Here's how the part is built. I have some questions about the finished solid (model axes, mm). Face numbers are marked on the shaded views. A direction names the side the tool comes from. Give positions to 0.01 mm unless a question says otherwise; leave off trailing zeros. Loops run counter-clockwise (first coordinate to the right, second up) from the corner with the lowest first, then second, coordinate; pieces in that order, holes last. Notation, with made-up numbers: (56, -26.75) - (109, -26.75) arc R36 cw to (109, 7.25) - close; hole circle Ø4 at (13.25, 10). An arc over 180 degrees is marked (long way). Return JSON: item names as keys, results as strings. Group by question number.
(1) I need wall thicknesses on probe 1 along X at (y, z) = (20, 17); probe 2 along X at (y, z) = (52, 0); probe 3 along Y at (x, z) = (-4.5, -24). Which ranges of each line are inside material? Lowest first, please. Write a range as [from, to].
(2) For P1, Ø3.5, axis at x = 0.5, y = 47.5, coming from the -Z side; P2, Ø6, axis at x = 5.5, z = -25.5, coming from the -Y side; P3, Ø4, axis at x = -14.5, y = 11.5, coming from the -Z side, each with a flat end and sliding along its axis, tell me the tip position at first contact or that it passes through.
(3) If we section it at C-C (y = 32): Please give me the cut outline in (x, z).
(4) If we mould it in two halves opening along Z, with no side actions, what happens to the marked faces 1, 2, 3 and 4? For each: released by +Z, released by -Z, zero draft, split by the parting line, or undercut.
(5) If we section it at A-A (x = -1.5): Please give me the cut outline in (y, z).
(6) If we section it at B-B (z = 16): Please give me the cut outline in (x, y), then the cut area to 3 significant figures.
(7) If we section it at D-D (y = 71): Please give me the cut outline in (x, z), then the cut area to 3 significant figures.
(8) On a 3-axis mill with a long thin cutter (end or side, diameter ignored), from which of +Z, -Z, +X, -X, +Y, -Y can I reach the whole of each face in a straight line? I mean the marked faces 5, 6, 7, 8 and 9. Say none if no direction works.
```python
from build123d import *

# Parameters (mm, degrees)
SKETCH1_W               = 49
SKETCH1_H               = 49
SKETCH1_R               = 3.25
BOSS_EXTRUDE1_DEPTH     = 53
SKETCH2_W               = 44
SKETCH2_H               = 44
CUT_EXTRUDE1_DEPTH      = 47
SKETCH3_R               = 13
CUT_EXTRUDE2_DEPTH      = 2
CUT_EXTRUDE3_DEPTH      = 10
BOSS_EXTRUDE2_DEPTH     = 30
SKETCH7_W               = 20.5
SKETCH7_H               = 21
CUT_EXTRUDE6_DEPTH      = 59
CUT_EXTRUDE7_DEPTH      = 59
CUT_EXTRUDE7_DEPTH_BACK = 3
SKETCH10_R              = 2.75
CUT_EXTRUDE8_DEPTH      = 59
FILLET1_R               = 30
CUT_EXTRUDE9_DEPTH      = 50.0000001


with BuildPart() as part:
    # Sketch1 → Boss-Extrude1 (new body)
    with BuildSketch(Plane(origin=(0, 0, 0), x_dir=(1, 0, 0), z_dir=(0, 1, 0))):
        Rectangle(SKETCH1_W, SKETCH1_H)
        Circle(SKETCH1_R, mode=Mode.SUBTRACT)
    extrude(amount=BOSS_EXTRUDE1_DEPTH)

    # Sketch2 → Cut-Extrude1 (cut)
    with BuildSketch(Plane.XZ):
        Rectangle(SKETCH2_W, SKETCH2_H)
    extrude(amount=-CUT_EXTRUDE1_DEPTH, mode=Mode.SUBTRACT)

    # Sketch3 → Cut-Extrude2 (cut)
    with BuildSketch(Plane.XZ.offset(-47)):
        Circle(SKETCH3_R)
    extrude(amount=-CUT_EXTRUDE2_DEPTH, mode=Mode.SUBTRACT)

    # Sketch4 → Cut-Extrude3 (cut)
    with BuildSketch(Plane(origin=(0, 53, 0), x_dir=(1, 0, 0), z_dir=(0, 1, 0))):
        with BuildLine():
            Line((-14.86862915, 17.13137085), (-11.36862915, 13.63137085))
            ThreePointArc((-11.36862915, 13.63137085), (-11.36862915, 11.36862915), (-13.63137085, 11.36862915))
            Line((-13.63137085, 11.36862915), (-17.13137085, 14.86862915))
            ThreePointArc((-17.13137085, 14.86862915), (-17.13137085, 17.13137085), (-14.86862915, 17.13137085))
        make_face()
        with BuildLine():
            Line((11.36862915, 13.63137085), (14.86862915, 17.13137085))
            ThreePointArc((14.86862915, 17.13137085), (17.13137085, 17.13137085), (17.13137085, 14.86862915))
            Line((17.13137085, 14.86862915), (13.63137085, 11.36862915))
            ThreePointArc((13.63137085, 11.36862915), (11.36862915, 11.36862915), (11.36862915, 13.63137085))
        make_face()
        with BuildLine():
            Line((13.63137085, -11.36862915), (17.13137085, -14.86862915))
            ThreePointArc((17.13137085, -14.86862915), (17.13137085, -17.13137085), (14.86862915, -17.13137085))
            Line((14.86862915, -17.13137085), (11.36862915, -13.63137085))
            ThreePointArc((11.36862915, -13.63137085), (11.36862915, -11.36862915), (13.63137085, -11.36862915))
        make_face()
        with BuildLine():
            Line((-11.36862915, -13.63137085), (-14.86862915, -17.13137085))
            ThreePointArc((-14.86862915, -17.13137085), (-17.13137085, -17.13137085), (-17.13137085, -14.86862915))
            Line((-17.13137085, -14.86862915), (-13.63137085, -11.36862915))
            ThreePointArc((-13.63137085, -11.36862915), (-11.36862915, -11.36862915), (-11.36862915, -13.63137085))
        make_face()
    extrude(amount=-CUT_EXTRUDE3_DEPTH, mode=Mode.SUBTRACT)

    # Sketch5 → Boss-Extrude2 (add)
    with BuildSketch(Plane(origin=(0, 53, 0), x_dir=(1, 0, 0), z_dir=(0, 1, 0))):
        with BuildLine():
            Line((-20.5, -24.5), (-12.942531675, 1.221013453))
            ThreePointArc((-12.942531675, 1.221013453), (-8.750052146, 9.614394804), (0, 13))
            ThreePointArc((0, 13), (8.750052146, 9.614394804), (12.942531675, 1.221013453))
            Line((12.942531675, 1.221013453), (20.5, -24.5))
            Line((20.5, -24.5), (24.5, -24.5))
            Line((24.5, -24.5), (24.5, 35))
            Line((24.5, 35), (-24.5, 35))
            Line((-24.5, 35), (-24.5, -24.5))
            Line((-24.5, -24.5), (-20.5, -24.5))
        make_face()
    extrude(amount=BOSS_EXTRUDE2_DEPTH)

    # Sketch7 → Cut-Extrude6 (cut)
    with BuildSketch(Plane.ZY.offset(24.5)):
        with Locations((-24.75, 63.5)):
            Rectangle(SKETCH7_W, SKETCH7_H)
    extrude(amount=-CUT_EXTRUDE6_DEPTH, mode=Mode.SUBTRACT)

    # Sketch9 → Cut-Extrude7 (cut, two sides)
    with BuildSketch(Plane(origin=(0, 53, 0), x_dir=(1, 0, 0), z_dir=(0, 1, 0))) as cut_extrude7_sk:
        with BuildLine():
            Line((-14.621320344, 10.378679656), (-18.121320344, 13.878679656))
            ThreePointArc((-18.121320344, 13.878679656), (-18.121320344, 18.121320344), (-13.878679656, 18.121320344))
            Line((-13.878679656, 18.121320344), (-10.378679656, 14.621320344))
            ThreePointArc((-10.378679656, 14.621320344), (-10.378679656, 10.378679656), (-14.621320344, 10.378679656))
        make_face()
        with BuildLine():
            Line((10.378679656, 14.621320344), (13.878679656, 18.121320344))
            ThreePointArc((13.878679656, 18.121320344), (18.121320344, 18.121320344), (18.121320344, 13.878679656))
            Line((18.121320344, 13.878679656), (14.621320344, 10.378679656))
            ThreePointArc((14.621320344, 10.378679656), (10.378679656, 10.378679656), (10.378679656, 14.621320344))
        make_face()
        with BuildLine():
            Line((13.878679656, -18.121320344), (10.378679656, -14.621320344))
            ThreePointArc((10.378679656, -14.621320344), (10.378679656, -10.378679656), (14.621320344, -10.378679656))
            Line((14.621320344, -10.378679656), (18.121320344, -13.878679656))
            ThreePointArc((18.121320344, -13.878679656), (18.121320344, -18.121320344), (13.878679656, -18.121320344))
        make_face()
        with BuildLine():
            Line((-13.878679656, -18.121320344), (-10.378679656, -14.621320344))
            ThreePointArc((-10.378679656, -14.621320344), (-10.378679656, -10.378679656), (-14.621320344, -10.378679656))
            Line((-14.621320344, -10.378679656), (-18.121320344, -13.878679656))
            ThreePointArc((-18.121320344, -13.878679656), (-18.121320344, -18.121320344), (-13.878679656, -18.121320344))
        make_face()
    extrude(amount=CUT_EXTRUDE7_DEPTH, mode=Mode.SUBTRACT)
    extrude(cut_extrude7_sk.sketch, amount=-CUT_EXTRUDE7_DEPTH_BACK, mode=Mode.SUBTRACT)

    # Sketch10 → Cut-Extrude8 (cut)
    with BuildSketch(Plane.XZ.offset(-74)):
        with Locations((14.5, -24.5)):
            Circle(SKETCH10_R)
        with Locations((-14.5, -24.5)):
            Circle(SKETCH10_R)
    extrude(amount=-CUT_EXTRUDE8_DEPTH, mode=Mode.SUBTRACT)

    # Fillet1
    fillet1_edges = [part.edges().sort_by_distance(p)[0] for p in [
        (22.5, 83, 24.5),
        (-22.5, 83, 24.5),
    ]]
    fillet(fillet1_edges, radius=FILLET1_R)

    # Sketch11 → Cut-Extrude9 (cut, through all)
    with BuildSketch(Plane(origin=(24.5, 0, 0), x_dir=(0, 0, -1), z_dir=(1, 0, 0))):
        Polygon((24.5, 0), (24.5, 42), (22, 42), (-22, 0), align=None)
    extrude(amount=-CUT_EXTRUDE9_DEPTH, mode=Mode.SUBTRACT)


solid = part.part
```
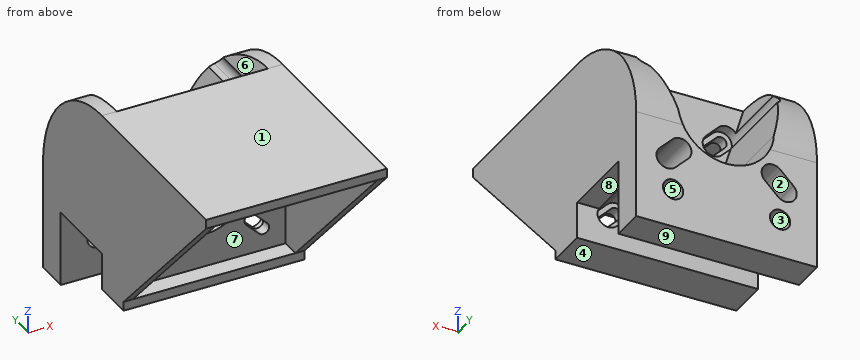
Values:
{
 "1": {"probe 1": "[-24.5, -22], [22, 24.5]", "probe 2": "[-24.5, -3.25], [3.25, 24.5]", "probe 3": "[42, 53], [74, 83]"},
 "2": {"P1": "z = -24.5", "P2": "y = 42", "P3": "z = 22"},
 "3": {"outline": "(-24.5, -11.52) - (-22, -11.52) - (-22, 22) - (22, 22) - (22, -11.52) - (24.5, -11.52) - (24.5, 24.5) - (-24.5, 24.5) - close"},
 "4": {"face 1": "released by +Z", "face 2": "undercut", "face 3": "undercut", "face 4": "released by -Z"},
 "5": {"outline": "(0, 22) - (47, 22) - (47, 12.91) - (49, 12.91) - (49, 2.88) - (53, 2.88) - (53, 24.5) - (0, 24.5) - close; (42, -24.5) - (53, -24.5) - (53, -14.5) - (74, -14.5) - (74, -35) - (83, -35) - (83, -12.91) - (53, -12.91) - (53, -2.88) - (49, -2.88) - (49, -12.91) - (47, -12.91) - (47, -22) - (42, -22) - close"},
 "6": {"outline": "(-24.5, 5.73) - (-22, 5.73) - (-22, 47) - (-17.6, 47) - (-17.6, 50) - (-19, 50) - (-19, 73.92) - (-24.5, 73.92) - close; (-13.74, 47) - (13.74, 47) - (13.74, 50) - (11.76, 50) - (11.76, 53) - (-11.76, 53) - (-11.76, 50) - (-13.74, 50) - close; (17.6, 47) - (22, 47) - (22, 5.73) - (24.5, 5.73) - (24.5, 73.92) - (19, 73.92) - (19, 50) - (17.6, 50) - close", "area": "664 mm2"},
 "7": {"outline": "(-24.5, -14.5) - (-18.6, -14.5) arc R3 cw to (-18.12, -13.88) - (-14.62, -10.38) arc R3 cw to (-10.26, -14.5) - (10.26, -14.5) arc R3 cw to (14.62, -10.38) - (18.12, -13.88) arc R3 cw to (18.6, -14.5) - (24.5, -14.5) - (24.5, 18.5) - (18.74, 18.5) - (18.49, 17.67) arc R3 cw to (18.12, 13.88) - (17.07, 12.83) - (12.94, -1.22) arc R13 cw to (-12.94, -1.22) - (-17.07, 12.83) - (-18.12, 13.88) arc R3 cw to (-18.49, 17.67) - (-18.74, 18.5) - (-24.5, 18.5) - close", "area": "689 mm2"},
 "8": {"face 5": "+Y", "face 6": "+Z, +Y", "face 7": "-Y", "face 8": "-Z, +X, -X", "face 9": "-Z, +X, -X, +Y, -Y"}
}
